```python
from build123d import *

# Parameters (mm, degrees)
F1_DEPTH = 2.032
F2_DEPTH = 1


# Not quite as in the source:
# - a feature names something its author has since deleted; it is built from what else it names


with BuildPart() as f1:
    # F0 (on Front) → F1 (new body)
    with BuildSketch(Plane.XZ):
        Polygon((-15.2212520439, 36.2265945869), (-17.3485020439, 36.2265945869), (-19.4757520439, 36.2265945869), (-19.4757520439, 34.1818945869), (-21.6982520439, 34.1818945869), (-21.6982520439, 31.9593945869), (-23.7429520439, 31.9593945869), (-23.7429520439, 29.8321445869), (-23.7429520439, 27.7048945869), (-21.6982520439, 27.7048945869), (-21.6982520439, 25.4823945869), (-19.4757520439, 25.4823945869), (-19.4757520439, 23.4376945869), (-17.3485020439, 23.4376945869), (-15.2212520439, 23.4376945869), (-15.2212520439, 25.4823945869), (-12.9987520439, 25.4823945869), (-12.9987520439, 27.7048945869), (-10.9540520439, 27.7048945869), (-10.9540520439, 29.8321445869), (-10.9540520439, 31.9593945869), (-12.9987520439, 31.9593945869), (-12.9987520439, 34.1818945869), (-15.2212520439, 34.1818945869), align=None)
        Polygon((-20.2887904064, 26.8476658233), (-17.9100000431, 32.8906836652), (-17.3217338641, 32.8878096037), (-14.9560986218, 26.8476658233), (-15.6798228753, 26.8476658233), (-16.4316139315, 28.7639858865), (-18.8453636264, 28.7639858865), (-19.5791117047, 26.8476658233), align=None, mode=Mode.SUBTRACT)
        Polygon((-17.3217338641, 32.8878096037), (-17.9100000431, 32.8906836652), (-20.2887904064, 26.8476658233), (-19.5791117047, 26.8476658233), (-18.8453636264, 28.7639858865), (-16.4316139315, 28.7639858865), (-15.6798228753, 26.8476658233), (-14.9560986218, 26.8476658233), align=None)
        Polygon((-18.5900452678, 29.3939520338), (-17.6306684633, 32.1173264378), (-16.6415135508, 29.3939520338), align=None, mode=Mode.SUBTRACT)
        Polygon((-16.6415135508, 29.3939520338), (-17.6306684633, 32.1173264378), (-18.5900452678, 29.3939520338), align=None)
    extrude(amount=F1_DEPTH)

    # F0 (on Front) → F2 (cut)
    with BuildSketch(Plane.XZ):
        Polygon((-17.3217338641, 32.8878096037), (-17.9100000431, 32.8906836652), (-20.2887904064, 26.8476658233), (-19.5791117047, 26.8476658233), (-18.8453636264, 28.7639858865), (-16.4316139315, 28.7639858865), (-15.6798228753, 26.8476658233), (-14.9560986218, 26.8476658233), align=None)
        Polygon((-18.5900452678, 29.3939520338), (-17.6306684633, 32.1173264378), (-16.6415135508, 29.3939520338), align=None, mode=Mode.SUBTRACT)
    extrude(amount=F2_DEPTH, mode=Mode.SUBTRACT)


solid = f1.part
```
Verification items for the finished model (mm, model axes). A direction names the side the tool comes from. Give positions to 0.01 mm unless a question says otherwise; leave off trailing zeros. Order: outer loops, then holes, each group sorted by start corner. A loop starts at its lowest first (then second) coordinate and runs counter-clockwise, first axis right, second up. Notation, with made-up numbers: (25.25, 59.5) - (75.25, 59.5) arc R21 cw to (75.25, 84.5) - close; hole circle Ø3 at (48.25, 79). An arc over 180 degrees is marked (long way). Answer as CSV lines item,"result". Start each with the question number.
Item 1: Section check B-B, the plane y = -1.45. Record the boundary of the cut face in (x, z).
Item 2: Material ranges on L1, parallel to X at y = -0.8, z = 27; L2, parallel to X at y = -0.95, z = 27.5; L3, parallel to X at y = -0.9, z = 35.25, recorded low to high.
Item 3: Mould release check, pull along Z, two halves, no side actions. Record for faces 6 (the face through (-18.117, -0.493, 30.737)), 7 (the face through (-17.6, -0.5, 29.394)), 8 (the face through (-19.476, -1, 24)), 9 (the face through (-17, -1, 23.438)): released by +Z, released by -Z, zero draft, split by the parting line, or undercut.
Item 4: Section check C-C, the plane z = 34.5. Record the boundary of the cut face in (x, y).
Item 5: Section check A-A, the plane y = -0.65. State how many separate pieces and enclosed holes the cut face has, plus the area to 3 significant figures.
Item 6: Access from +Z, -Z, +X, -X, +Y, -Y to the whole of each face (thin tool, end or side, straight path). Record for faces 1 (the face through (-15.221, -1, 24)), 2 (the face through (-14, -1, 34.182)), 3 (the face through (-17.14, -0.49, 30.77)), 4 (the face through (-17, -1, 36.227)), 5 (the face through (-21.698, -1, 27)).
Item 7: Section check D-D, the plane x = -16. Record the boundary of the cut face in (y, z).
Item 8: Gauge pin test, flat ends, axial feed: pin 1 (4.5 mm diameter, centred on x = -16.5, z = 29, fed in from +Y); pin 2 (0.6 mm diameter, centred on x = -11.5, y = -1.5, fed in from +Z); pin 3 (0.8 mm diameter, centred on x = -20, y = -0.5, fed in from +Z); pin 4 (0.6 mm diameter, centred on x = -13.5, y = -1, fed in from -Z). Record the tip position at first contact, or that the pin passes through.
Filled in:
1,outline,"(-23.74, 27.7) - (-21.7, 27.7) - (-21.7, 25.48) - (-19.48, 25.48) - (-19.48, 23.44) - (-15.22, 23.44) - (-15.22, 25.48) - (-13, 25.48) - (-13, 27.7) - (-10.95, 27.7) - (-10.95, 31.96) - (-13, 31.96) - (-13, 34.18) - (-15.22, 34.18) - (-15.22, 36.23) - (-19.48, 36.23) - (-19.48, 34.18) - (-21.7, 34.18) - (-21.7, 31.96) - (-23.74, 31.96) - close"
2,L1,"-21.7 to -20.23, -19.52 to -15.74, -15.02 to -13"
2,L2,"-21.7 to -20.03, -19.33 to -15.94, -15.21 to -13"
2,L3,"-19.48 to -15.22"
3,face 6,"undercut"
3,face 7,"undercut"
3,face 8,"zero draft"
3,face 9,"released by -Z"
4,outline,"(-19.48, -2.03) - (-15.22, -2.03) - (-15.22, 0) - (-19.48, 0) - close"
5,separate pieces,"2"
5,enclosed holes,"1"
5,area,"101 mm^2"
6,face 1,"-Z, +X, +Y, -Y"
6,face 2,"+Z, +X, +Y, -Y"
6,face 3,"+Y"
6,face 4,"+Z, +X, -X, +Y, -Y"
6,face 5,"-Z, -X, +Y, -Y"
7,outline,"(-2.03, 23.44) - (0, 23.44) - (0, 27.66) - (-1, 27.66) - (-1, 29.51) - (0, 29.51) - (0, 36.23) - (-2.03, 36.23) - close"
8,pin 1,"y = 0"
8,pin 2,"z = 31.96"
8,pin 3,"z = 34.18"
8,pin 4,"z = 25.48"
